Design review of the part shown in the three views and the two pictorial views. Dimensions are in mm from the part's minimum x, y and z. A direction names the side the tool comes from. Round coordinates to 2 decimals unless told otherwise and drop trailing zeros. Write each loop counter-clockwise with the first axis right and the second up, starting at its lowest first coordinate (ties: lowest second). Pieces come first, ordered by that corner, then holes. Notation, with made-up numbers: (84.25, -18.5) -> (117.25, -18.5) arc R20 ccw to (117.25, -8.5) -> close; hole circle Ø7 at (60.5, 47.25). An arc over 180 degrees is marked (long way). One line per question, with ' | ' between items. Start each with the question number.
1) Consider section B-B (y = 40). Give the boundary of the cut face in (x, z).
2) Consider section C-C (x = 36). Give the boundary of the cut face in (y, z).
3) For probe 1 along Y at (x, z) = (40, 27.2); probe 2 along X at (y, z) = (74.5, 18), list the stretches that pass through material, from the lowest coordinate up.
4) Consider section D-D (y = 13). Give the boundary of the cut face in (x, z), then the cut area to 3 significant figures.
5) Consider section A-A (z = 12). Give the boundary of the cut face in (x, y).
6) For the marked faces 1 and 2, list the 3-axis set-ups (+Z, -Z, +X, -X, +Y, -Y) from which the entire face can be reached by the end or side of a thin tool; tool diameter is ignored.
7) Mouldability with a two-part tool opening along X and no side actions: class the marked faces 3, 4 and 5 as +X half, -X half, draft (parallel to the pull), parting line (faces both ways), or undercut.
8) Insertion check: pin 1 Ø8 at (x, y) = (16.5, 61) entering from -Z. The pin has a flat end and moves straight along its axis. Give the tip position at first contact, or say it passes through.
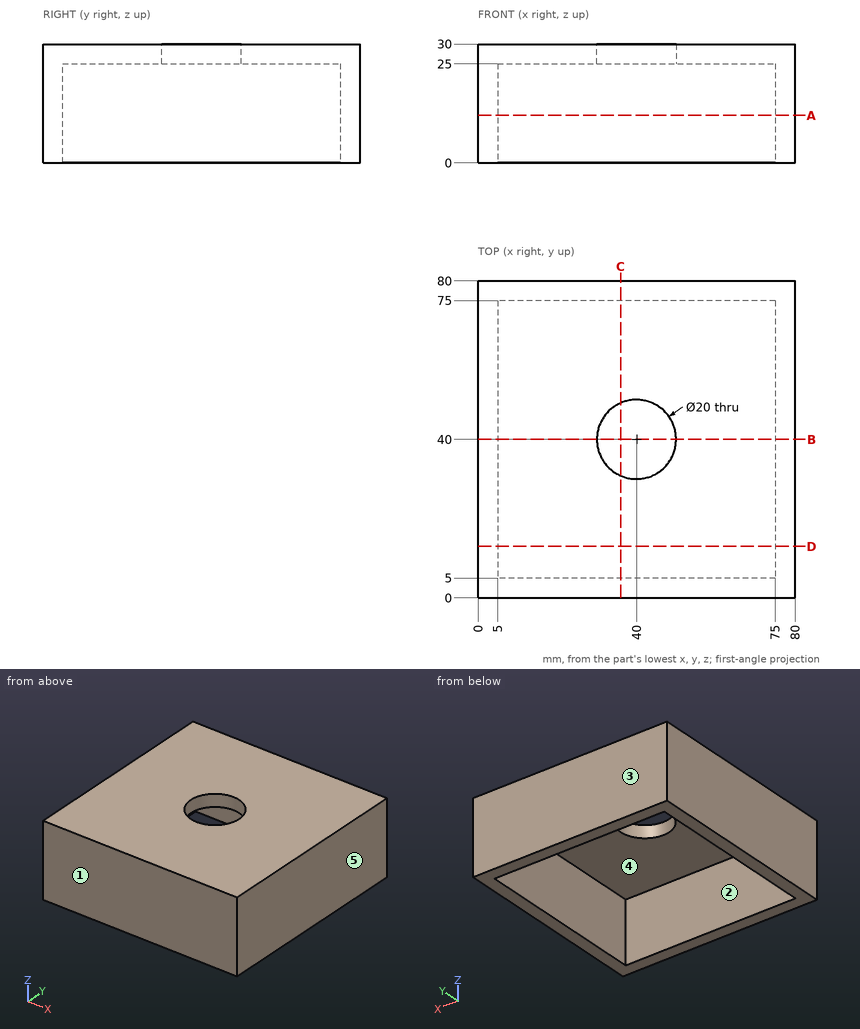
From the geometry:
1) outline: (0, 0) -> (5, 0) -> (5, 25) -> (30, 25) -> (30, 30) -> (0, 30) -> close; (50, 25) -> (75, 25) -> (75, 0) -> (80, 0) -> (80, 30) -> (50, 30) -> close
2) outline: (0, 0) -> (5, 0) -> (5, 25) -> (30.83, 25) -> (30.83, 30) -> (0, 30) -> close; (49.17, 25) -> (75, 25) -> (75, 0) -> (80, 0) -> (80, 30) -> (49.17, 30) -> close
3) probe 1: y = 0 to 30, 50 to 80 | probe 2: x = 0 to 5, 75 to 80
4) outline: (0, 0) -> (5, 0) -> (5, 25) -> (75, 25) -> (75, 0) -> (80, 0) -> (80, 30) -> (0, 30) -> close | area: 650 mm2
5) outline: (0, 0) -> (80, 0) -> (80, 80) -> (0, 80) -> close; hole (5, 5) -> (75, 5) -> (75, 75) -> (5, 75) -> close
6) face 1: +Z, -Z, +X, -X, -Y | face 2: -Z
7) face 3: draft | face 4: undercut | face 5: +X half
8) pin 1: stops at z = 25
